from build123d import *

# Parameters (mm, degrees)
SKETCH_1_W      = 0.7
SKETCH_1_H      = 1.5
EXTRUDE_1_DEPTH = 0.2


with BuildPart() as part:
    # 스케치1 → 보스-돌출1 (new body)
    with BuildSketch(Plane.XZ):
        Polygon((28.47, -5.1), (24.77, -8.8), (15.23, -8.8), (11.53, -5.1), (11.53, -2.8), (28.47, -2.8), align=None)
        with Locations((12.38, -3.75)):
            Rectangle(SKETCH_1_W, SKETCH_1_H, mode=Mode.SUBTRACT)
        with Locations((13.65, -3.75)):
            Rectangle(SKETCH_1_W, SKETCH_1_H, mode=Mode.SUBTRACT)
        with Locations((14.92, -3.75)):
            Rectangle(SKETCH_1_W, SKETCH_1_H, mode=Mode.SUBTRACT)
        with Locations((16.19, -3.75)):
            Rectangle(SKETCH_1_W, SKETCH_1_H, mode=Mode.SUBTRACT)
        with Locations((17.46, -3.75)):
            Rectangle(SKETCH_1_W, SKETCH_1_H, mode=Mode.SUBTRACT)
        with Locations((18.73, -3.75)):
            Rectangle(SKETCH_1_W, SKETCH_1_H, mode=Mode.SUBTRACT)
        with Locations((20, -3.75)):
            Rectangle(SKETCH_1_W, SKETCH_1_H, mode=Mode.SUBTRACT)
        with Locations((21.27, -3.75)):
            Rectangle(SKETCH_1_W, SKETCH_1_H, mode=Mode.SUBTRACT)
        with Locations((22.54, -3.75)):
            Rectangle(SKETCH_1_W, SKETCH_1_H, mode=Mode.SUBTRACT)
        with Locations((23.81, -3.75)):
            Rectangle(SKETCH_1_W, SKETCH_1_H, mode=Mode.SUBTRACT)
        with Locations((25.08, -3.75)):
            Rectangle(SKETCH_1_W, SKETCH_1_H, mode=Mode.SUBTRACT)
        with Locations((26.35, -3.75)):
            Rectangle(SKETCH_1_W, SKETCH_1_H, mode=Mode.SUBTRACT)
        with Locations((27.62, -3.75)):
            Rectangle(SKETCH_1_W, SKETCH_1_H, mode=Mode.SUBTRACT)
    extrude(amount=EXTRUDE_1_DEPTH)


solid = part.part
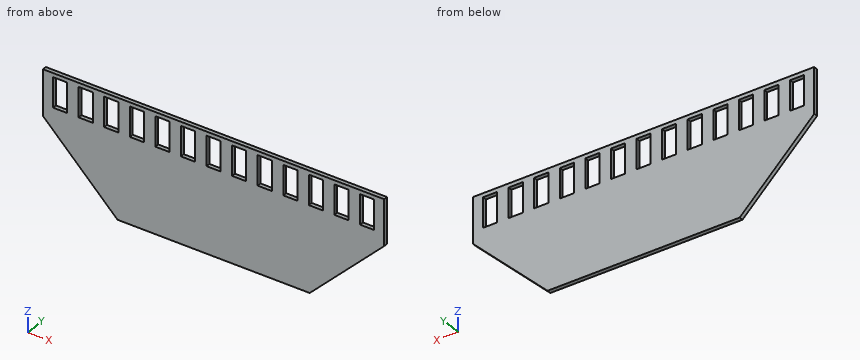
Can you work these out from the model? Positions are in its coordinate system, mm. Give positions to 0.01 mm unless a question says otherwise; leave off trailing zeros. Loops run counter-clockwise (first coordinate to the right, second up) from the corner with the lowest first, then second, coordinate; pieces in that order, holes last. Notation, with made-up numbers: (-11.5, 29) -> (41.5, 29) arc R24 ccw to (41.5, 48) -> close; hole circle Ø8 at (88.5, 61.25). An arc over 180 degrees is marked (long way). Return JSON: item names as keys, results as strings.
Q1. I want a section at A-A, the plane z = -3.5. Count the separate pieces of the cut face and the enclosed holes in it, then the cut area to 3 significant figures.
Checks:
{"separate pieces": "14", "enclosed holes": "0", "area": "1.57 mm2"}
Q2. I want a section at B-B, the plane z = -8.25. List the corners of the cut face in (x, y) for me.
Checks:
{"outline": "(14.68, -0.2) -> (25.32, -0.2) -> (25.32, 0) -> (14.68, 0) -> close"}
Q3. I want a section at D-D, the plane z = -7.5. List the corners of the cut face in (x, y) for me, then the cut area to 3 significant figures.
Checks:
{"outline": "(13.93, -0.2) -> (26.07, -0.2) -> (26.07, 0) -> (13.93, 0) -> close", "area": "2.43 mm2"}
Q4. I need wall thicknesses on probe 1 along Z at (x, y) = (23.5, -0.1); probe 2 along X at (y, z) = (-0.1, -7); probe 3 along X at (y, z) = (-0.1, -6). Which ranges of each line are inside material? Lowest first, please.
Checks:
{"probe 1": "z = -8.8 to -4.5, -3 to -2.8", "probe 2": "x = 13.43 to 26.57", "probe 3": "x = 12.43 to 27.57"}
